Here's how the part is built. I have some questions about the finished solid (model axes, mm). A direction names the side the tool comes from. Round coordinates to 2 decimals unless told otherwise and drop trailing zeros. Order: outer loops, then holes, each group sorted by start corner. A loop starts at its lowest first (then second) coordinate and runs counter-clockwise, first axis right, second up. Notation, with made-up numbers: M -14,-14.5 L 6,-14.5 A27 cw 6,19.5 Z; hole C 47,34 d11. An arc over 180 degrees is marked long. Write item = value, one per line. Start each with the question number.
Item 1: I want a section at C-C, the plane y = -17. List the corners of the cut face in (x, z) for me.
Item 2: We'd pull the mould along X, two halves only. Please class faces 3 (the face through (0.33, -21.172, -7.493)), 4 (the face through (3.15, -20, 0)): pulls with the +X half, pulls with the -X half, needs draft (parallel to the pull), parting line crosses it, or undercut.
Item 3: I want a section at B-B, the plane y = -3.5. List the corners of the cut face in (x, z) for me, plus the area to 3 significant figures.
Item 4: For faces 1 (the face through (0, -20, -3.15)), 2 (the face through (3.3, -8.1, -5.6)), which set-ups out of +Z, -Z, +X, -X, +Y, -Y let a thin tool reach every point of the face, with its end or its side?
Item 5: I'm going to push flat-ended pins straight in: P1, Ø4, axis at y = -18.5, z = -5, coming from the +X side; P2, Ø3, axis at x = -1, y = -19.5, coming from the +Z side; P3, Ø6, axis at x = -4, y = -7, coming from the -Z side. Where does each tip first touch, or does it pass through?
Item 6: Please list where these lines run through material, in increasing order: L1, parallel to X at y = -4.75, z = 3.25; L2, parallel to Y at x = -3.75, z = -3.5; L3, parallel to Z at x = 2.75, y = -14.
Item 7: I want a section at A-A, the plane z = 0. List the corners of the cut face in (x, y) for me.
Solid Edge part; units mm, degrees
sketch "Sketch1" plane through (0, 0, 0) normal (1, 0, 0) x (0, 1, 0)
  line L0 (-25, 7.5) -> (-16, 7.5)
  line L1 (-16, 7.5) -> (-16, 9)
  line L2 (-16, 9) -> (0, 9)
  line L3 (0, 9) -> (0, 0)
  line L4 (-25, 0) -> (-25, 7.5)
  dimension "D1" = 16
revolve "RevolvedProtrusion1" add sketch "Sketch1" angle 360 about axis through (0, 0, 0) along (0, -1, 0)
sketch "Sketch2" plane through (0, 0, 0) normal (0, 1, 0) x (-1, 0, 0)
  line L0 (0, -7.5056) -> (6.5, -3.7528)
  line L1 (6.5, -3.7528) -> (6.5, 3.7528)
  line L2 (6.5, 3.7528) -> (0, 7.5056)
  line L3 (0, 7.5056) -> (-6.5, 3.7528)
  line L4 (-6.5, 3.7528) -> (-6.5, -3.7528)
  line L5 (-6.5, -3.7528) -> (0, -7.5056)
extrude "Cutout1" cut sketch "Sketch2" against normal blind 15.5
sketch "Sketch3" plane through (0, -25, 0) normal (0, -1, 0) x (1, 0, 0)
  line L0 (3.15, 3.15) -> (-3.15, 3.15)
  line L1 (-3.15, 3.15) -> (-3.15, -3.15)
  line L2 (-3.15, -3.15) -> (3.15, -3.15)
  line L3 (3.15, -3.15) -> (3.15, 3.15)
  dimension "D1" = 3.15
extrude "Extrusionsausschnitt_2" cut sketch "Sketch3" against normal blind 51.1789
fillet "Verrundung_1" radius 0.5 2 edges at (0, -25, 7.5) (0, 0, 9)
fillet "Verrundung_2" radius 2 1 edges at (0, -16, 7.5)
sketch "Sketch4" plane through (0, 0, 0) normal (1, 0, 0) x (0, 1, 0)
  line L0 (0, -8) -> (-13.8564, 0)
  line L1 (0, 0) -> (0, -8)
revolve "RevolvedCutout1" cut sketch "Sketch4" angle 360 about axis through (0, 0, 0) along (0, -1, 0)
Filled in:
q1.outline = C 0,0 d15.47; hole M -3.15,-3.15 L 3.15,-3.15 L 3.15,3.15 L -3.15,3.15 Z
q2.face_3 = parting line crosses it
q2.face_4 = undercut
q3.outline = C 0,0 d18; hole M -6.5,-3.75 L 0,-7.51 L 6.5,-3.75 L 6.5,3.75 L 0,7.51 L -6.5,3.75 Z
q3.area = 108 mm^2
q4.face_1 = +Y, -Y
q4.face_2 = +Y
q5.P1 = 6.87
q5.P2 = 7.5
q5.P3 = -8.94
q6.L1 = -8.39 to -6.5, 6.5 to 8.39
q6.L2 = -25 to -15.5
q6.L3 = -8.57 to -5.92, 5.92 to 8.57
q7.outline = M -9,-16 A2 cw -7.5,-17.94 L -7.5,-24.5 A0.5 ccw -7,-25 L -3.15,-25 L -3.15,-15.5 L -6.5,-15.5 L -6.5,-2.6 L -8,0 L -8.5,0 A0.5 ccw -9,-0.5 Z; M 3.15,-25 L 7,-25 A0.5 ccw 7.5,-24.5 L 7.5,-17.94 A2 cw 9,-16 L 9,-0.5 A0.5 ccw 8.5,0 L 8,0 L 6.5,-2.6 L 6.5,-15.5 L 3.15,-15.5 Z
